from build123d import *

# Parameters (mm, degrees)
SKETCH1_W                                           = 50.8
SKETCH1_H                                           = 76.2
BOSS_EXTRUDE1_DEPTH                                 = 12.7
CSK_FOR_M4_FLAT_HEAD_MACHINE_SCREW1_D               = 4.5
CSK_FOR_M4_FLAT_HEAD_MACHINE_SCREW1_CSINK_D         = 9.4
CSK_FOR_M4_FLAT_HEAD_MACHINE_SCREW1_CSINK_ANGLE     = 90
CBORE_FOR_8_BINDING_HEAD_MACHINE_SCREW1_D           = 4.4958
CBORE_FOR_8_BINDING_HEAD_MACHINE_SCREW1_CBORE_D     = 9.525
CBORE_FOR_8_BINDING_HEAD_MACHINE_SCREW1_CBORE_DEPTH = 2.667


with BuildPart() as part:
    # Sketch1 → Boss-Extrude1 (new body)
    with BuildSketch(Plane(origin=(0, 0, 0), x_dir=(0, 0, -1), z_dir=(1, 0, 0))):
        Rectangle(SKETCH1_W, SKETCH1_H)
    extrude(amount=BOSS_EXTRUDE1_DEPTH)

    # CSK for M4 Flat Head Machine Screw1 (through all)
    with Locations(Plane(origin=(12.7, 0, 0), x_dir=(0, 0, -1), z_dir=(1, 0, 0))):
        with Locations((11.136931804, 28.623863607), (-11.136931804, 28.623863607), (-11.136931804, 6.35), (11.136931804, 6.35)):
            CounterSinkHole(CSK_FOR_M4_FLAT_HEAD_MACHINE_SCREW1_D / 2, CSK_FOR_M4_FLAT_HEAD_MACHINE_SCREW1_CSINK_D / 2, counter_sink_angle=CSK_FOR_M4_FLAT_HEAD_MACHINE_SCREW1_CSINK_ANGLE)

    # CBORE for #8 Binding Head Machine Screw1 (through all)
    with Locations(Plane.ZY):
        with Locations((-19.05, -31.75), (0, -31.75), (19.05, -31.75)):
            CounterBoreHole(CBORE_FOR_8_BINDING_HEAD_MACHINE_SCREW1_D / 2, CBORE_FOR_8_BINDING_HEAD_MACHINE_SCREW1_CBORE_D / 2, CBORE_FOR_8_BINDING_HEAD_MACHINE_SCREW1_CBORE_DEPTH)


solid = part.part
Work out the finished part from the listing and answer in its coordinate system (mm). A direction names the side the tool comes from. Round coordinates to 2 decimals unless told otherwise and drop trailing zeros. Order: outer loops, then holes, each group sorted by start corner. A loop starts at its lowest first (then second) coordinate and runs counter-clockwise, first axis right, second up. Notation, with made-up numbers: M 38,44.5 L 50,44.5 A26 cw 50,71.5 Z; hole C -14,48.5 d5. An arc over 180 degrees is marked long. Put each result on its own line as item: value. Start each with the question number.
Q1. A tool of negligible diameter and unlimited length cuts with its end or side. For faces 4 (the cylindrical face through (1.31, -27.03, -0.62)), 5 (the cylindrical face through (7.754, -29.855, -1.208)), from which of +Z, -Z, +X, -X, +Y, -Y can it reach the whole face along a straight path? Write none if from no direction.
Q2. Section C-C, the plane y = 6.35 is taken. Write down the section's boundary in (x, z), and give its area (3 significant figures).
Q3. Section D-D, the plane x = 3.75 is taken. Write down the section's boundary in (y, z), and give its area (3 significant figures).
Q4. For a pull along Y with two mould halves and no side action, classify faces 1 (the flat face through (6, 38.1, 0)), 2 (the conical face through (10.37, 27.72, 13.33)), 3 (the flat face through (6, -1, 25.4)) as pulls with the +Y half, pulls with the -Y half, needs draft (parallel to the pull), parting line crosses it, or undercut.
Q5. Section B-B, the plane y = -31.75 is taken. Write down the section's boundary in (x, z).
Q6. Straight lines are drawn through the part: L1, parallel to Z at x = 7.5, y = 6.35; L2, parallel to Z at x = 10.5, y = -30; L3, parallel to Z at x = 3.5, y = -30.5. For each, find the intervals that lie inside material, in ascending order. Write a range as [from, to].
Q7. Flat-ended cylindrical pins translate along their axes: pin 1 (6 mm diameter, centred on y = -30, z = 1, fed in from -X); pin 2 (5 mm diameter, centred on y = -31.75, z = 0, fed in from -X). Find the tip coordinate at first contact, or state that the pin passes through.
Q8. Section A-A, the plane z = -19.05 is taken. Write down the section's boundary in (x, y).
Findings below:
1. face 4: -X
1. face 5: +X, -X
2. outline: M 0,-25.4 L 12.7,-25.4 L 12.7,-15.84 L 10.25,-13.39 L 0,-13.39 Z; M 0,-8.89 L 10.25,-8.89 L 12.7,-6.44 L 12.7,6.44 L 10.25,8.89 L 0,8.89 Z; M 0,13.39 L 10.25,13.39 L 12.7,15.84 L 12.7,25.4 L 0,25.4 Z
2. area: 519 mm^2
3. outline: M -38.1,-25.4 L 38.1,-25.4 L 38.1,25.4 L -38.1,25.4 Z; hole C -31.75,-19.05 d4.5; hole C -31.75,0 d4.5; hole C -31.75,19.05 d4.5; hole C 6.35,-11.14 d4.5; hole C 6.35,11.14 d4.5; hole C 28.62,-11.14 d4.5; hole C 28.62,11.14 d4.5
3. area: 3,760 mm^2
4. face 1: pulls with the +Y half
4. face 2: undercut
4. face 3: needs draft
5. outline: M 0,-25.4 L 12.7,-25.4 L 12.7,-21.3 L 2.67,-21.3 L 2.67,-23.81 L 0,-23.81 Z; M 0,-14.29 L 2.67,-14.29 L 2.67,-16.8 L 12.7,-16.8 L 12.7,-2.25 L 2.67,-2.25 L 2.67,-4.76 L 0,-4.76 Z; M 0,4.76 L 2.67,4.76 L 2.67,2.25 L 12.7,2.25 L 12.7,16.8 L 2.67,16.8 L 2.67,14.29 L 0,14.29 Z; M 0,23.81 L 2.67,23.81 L 2.67,21.3 L 12.7,21.3 L 12.7,25.4 L 0,25.4 Z
6. L1: z = [-25.4, -13.39], [-8.89, 8.89], [13.39, 25.4]
6. L2: z = [-25.4, -20.46], [-17.64, -1.41], [1.41, 17.64], [20.46, 25.4]
6. L3: z = [-25.4, -20.92], [-17.18, -1.87], [1.87, 17.18], [20.92, 25.4]
7. pin 1: stops at x = 0
7. pin 2: stops at x = 2.67
8. outline: M 0,-38.1 L 12.7,-38.1 L 12.7,-34 L 2.67,-34 L 2.67,-36.51 L 0,-36.51 Z; M 0,-26.99 L 2.67,-26.99 L 2.67,-29.5 L 12.7,-29.5 L 12.7,38.1 L 0,38.1 Z
